Here's how the part is built. I have some questions about the finished solid (model axes, mm). Face numbers are marked on the shaded views. A direction names the side the tool comes from. Give positions to 0.01 mm unless a question says otherwise; leave off trailing zeros. Order: outer loops, then holes, each group sorted by start corner. A loop starts at its lowest first (then second) coordinate and runs counter-clockwise, first axis right, second up.
from build123d import *

# Parameters (mm, degrees)
F1_DEPTH = 80
F2_R     = 3.3
F2_R_2   = 3
F3_DEPTH = 75.6
F4_R     = 3
F4_W     = 254.5
F4_H     = 154.5
F5_DEPTH = 66.6
F6_W     = 254.5
F6_H     = 154.5
F7_DEPTH = 9.4


with BuildPart() as f1:
    # F0 (on Top) → F1 (new body)
    with BuildSketch(Plane.XY):
        with BuildLine():
            Line((290, 0), (10, 0))
            ThreePointArc((10, 0), (2.928932, -2.928932), (0, -10))
            Line((0, -10), (0, -190))
            ThreePointArc((0, -190), (2.928932, -197.071068), (10, -200))
            Line((10, -200), (290, -200))
            ThreePointArc((290, -200), (297.071068, -197.071068), (300, -190))
            Line((300, -190), (300, -10))
            ThreePointArc((300, -10), (297.071068, -2.928932), (290, 0))
        make_face()
    extrude(amount=F1_DEPTH)

    # F2 (on face) → F3 (cut)
    with BuildSketch(Plane.XY.offset(80)):
        with Locations((10, -10)):
            Circle(F2_R)
        with Locations((10, -190)):
            Circle(F2_R)
        with Locations((290, -190)):
            Circle(F2_R)
        with Locations((290, -10)):
            Circle(F2_R)
        with Locations((16, -33)):
            Circle(F2_R_2)
        with Locations((16, -100)):
            Circle(F2_R_2)
        with Locations((16, -167)):
            Circle(F2_R_2)
        with Locations((284, -100)):
            Circle(F2_R_2)
        with Locations((284, -33)):
            Circle(F2_R_2)
        with Locations((284, -167)):
            Circle(F2_R_2)
    extrude(amount=-F3_DEPTH, mode=Mode.SUBTRACT)

    # F4 (on face) → F5 (cut)
    with BuildSketch(Plane.XY.offset(80)):
        with BuildLine():
            Line((274.288541, -6), (25.724985, -6))
            ThreePointArc((25.724985, -6), (23.537386, -6.947098), (22.731033, -9.190395))
            ThreePointArc((22.731033, -9.190395), (19.020384, -19.020384), (9.190395, -22.731033))
            ThreePointArc((9.190395, -22.731033), (6.947098, -23.537386), (6, -25.724985))
            Line((6, -25.724985), (6, -174.275015))
            ThreePointArc((6, -174.275015), (6.947098, -176.462614), (9.190395, -177.268967))
            ThreePointArc((9.190395, -177.268967), (19.020384, -180.979616), (22.731033, -190.809605))
            ThreePointArc((22.731033, -190.809605), (23.537386, -193.052902), (25.724985, -194))
            Line((25.724985, -194), (274.288541, -194))
            ThreePointArc((274.288541, -194), (276.476197, -193.052843), (277.282483, -190.809442))
            ThreePointArc((277.282483, -190.809442), (280.989161, -180.989161), (290.809442, -177.282483))
            ThreePointArc((290.809442, -177.282483), (293.052843, -176.476197), (294, -174.288541))
            Line((294, -174.288541), (294, -25.711459))
            ThreePointArc((294, -25.711459), (293.052843, -23.523803), (290.809442, -22.717517))
            ThreePointArc((290.809442, -22.717517), (280.989161, -19.010839), (277.282483, -9.190558))
            ThreePointArc((277.282483, -9.190558), (276.476197, -6.947157), (274.288541, -6))
        make_face()
        with Locations((16, -167)):
            Circle(F4_R, mode=Mode.SUBTRACT)
        with Locations((284, -167)):
            Circle(F4_R, mode=Mode.SUBTRACT)
        with Locations((16, -100)):
            Circle(F4_R, mode=Mode.SUBTRACT)
        with Locations((16, -33)):
            Circle(F4_R, mode=Mode.SUBTRACT)
        with Locations((150.00675, -100)):
            Rectangle(F4_W, F4_H, mode=Mode.SUBTRACT)
        with Locations((284, -100)):
            Circle(F4_R, mode=Mode.SUBTRACT)
        with Locations((284, -33)):
            Circle(F4_R, mode=Mode.SUBTRACT)
        with Locations((150.00675, -100)):
            Rectangle(F4_W, F4_H)
    extrude(amount=-F5_DEPTH, mode=Mode.SUBTRACT)

    # F6 (on face) → F7 (cut)
    with BuildSketch(Plane.XY.offset(13.4)):
        with Locations((150, -100)):
            Rectangle(F6_W, F6_H)
    extrude(amount=-F7_DEPTH, mode=Mode.SUBTRACT)


solid = f1.part
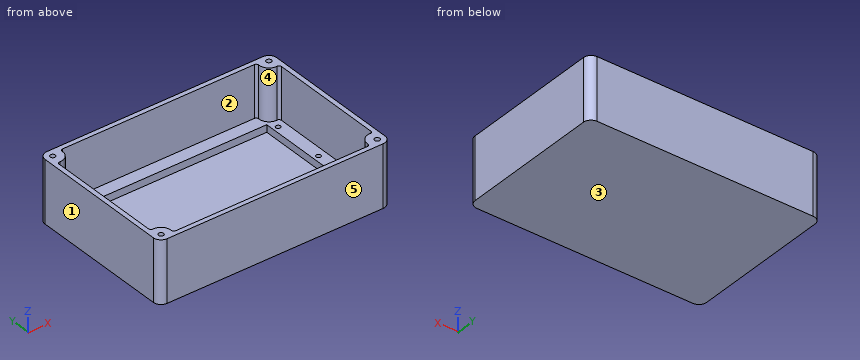
Q1. If we section it at D-D on y = -59: List the corners of the cut face in (x, z) for me.
Filled sheet:
outline: (0, 0) - (300, 0) - (300, 80) - (294, 80) - (294, 13.4) - (277.25, 13.4) - (277.25, 4) - (22.75, 4) - (22.75, 13.4) - (6, 13.4) - (6, 80) - (0, 80) - close
Q2. If we section it at B-B on y = -33: List the corners of the cut face in (x, z) for me.
Filled sheet:
outline: (0, 0) - (300, 0) - (300, 80) - (294, 80) - (294, 13.4) - (287, 13.4) - (287, 4.4) - (281, 4.4) - (281, 13.4) - (277.25, 13.4) - (277.25, 4) - (22.75, 4) - (22.75, 13.4) - (19, 13.4) - (19, 4.4) - (13, 4.4) - (13, 13.4) - (6, 13.4) - (6, 80) - (0, 80) - close
Q3. I need wall thicknesses on L1, parallel to X at y = -167, z = 7; L2, parallel to Y at x = 16, z = 8.75; L3, parallel to X at y = -190, z = 34. Which ranges of each line are inside material? Lowest first, please.
Filled sheet:
L1: x = 0 to 13, 19 to 22.75, 277.25 to 281, 287 to 300
L2: y = -200 to -170, -164 to -103, -97 to -36, -30 to 0
L3: x = 0 to 6.7, 13.3 to 22.76, 277.26 to 286.7, 293.3 to 300
Q4. For the marked faces 1 and 2, which set-ups out of +Z, -Z, +X, -X, +Y, -Y let a thin tool reach every point of the face, with its end or its side?
Filled sheet:
face 1: +Z, -Z, -X, +Y, -Y
face 2: +Z
Q5. If we section it at C-C on x = 242.5: List the corners of the cut face in (y, z) for me.
Filled sheet:
outline: (-200, 0) - (0, 0) - (0, 80) - (-6, 80) - (-6, 13.4) - (-22.75, 13.4) - (-22.75, 4) - (-177.25, 4) - (-177.25, 13.4) - (-194, 13.4) - (-194, 80) - (-200, 80) - close
Q6. If we section it at A-A on z = 50.5: List the corners of the cut face in (x, y) for me.
Filled sheet:
outline: (0, -190) arc R10 ccw to (10, -200) - (290, -200) arc R10 ccw to (300, -190) - (300, -10) arc R10 ccw to (290, 0) - (10, 0) arc R10 ccw to (0, -10) - close; hole (6, -174.28) arc R3 ccw to (9.19, -177.27) arc R12.76 cw to (22.73, -190.81) arc R3 ccw to (25.72, -194) - (274.29, -194) arc R3 ccw to (277.28, -190.81) arc R12.74 cw to (290.81, -177.28) arc R3 ccw to (294, -174.29) - (294, -25.71) arc R3 ccw to (290.81, -22.72) arc R12.74 cw to (277.28, -9.19) arc R3 ccw to (274.29, -6) - (25.72, -6) arc R3 ccw to (22.73, -9.19) arc R12.76 cw to (9.19, -22.73) arc R3 ccw to (6, -25.72) - close; hole circle Ø6.6 at (10, -190); hole circle Ø6.6 at (10, -10); hole circle Ø6.6 at (290, -190); hole circle Ø6.6 at (290, -10)
Q7. Thinking about a two-plate mould opening in Y: for the marked faces 3, 4 and 5, which applies, released by +Y, released by -Y, zero draft, split by the parting line, or undercut?
Filled sheet:
face 3: zero draft
face 4: undercut
face 5: released by -Y
Q8. I'm going to push flat-ended pins straight in: P1, Ø7.5, axis at x = 9.5, y = -191.5, coming from the +Z side; P2, Ø1.8, axis at x = 283, y = -31.5, coming from the +Z side; P3, Ø8, axis at x = 284, y = -100, coming from the +Z side; P4, Ø10, axis at x = 77.5, y = -33.5, coming from the +Z side. Where does each tip first touch, or does it pass through?
Filled sheet:
P1: stops at z = 80
P2: stops at z = 4.4
P3: stops at z = 13.4
P4: stops at z = 4
